Could you check a few things on this model? Use its own coordinates, in mm. Face numbers are marked on the shaded views. A direction names the side the tool comes from. Give positions to 0.01 mm unless a question says otherwise; leave off trailing zeros. Loops run counter-clockwise (first coordinate to the right, second up) from the corner with the lowest first, then second, coordinate; pieces in that order, holes last. Notation, with made-up numbers: M -3,-22 L 38,-22 A22 ccw 38,11 Z; hole C 23.25,16.25 d4. An arc over 180 degrees is marked long. Use CSV: the item, a comma, the result in double quotes.
```python
from build123d import *

# Parameters (mm, degrees)
F0_R     = 3.175
F1_DEPTH = 6.35
F2_R     = 1.8288
F3_R     = 1.8288
F4_DEPTH = 6.005883
F5_R     = 2.54


with BuildPart() as f1:
    # F0 (on Top) → F1 (new body)
    with BuildSketch(Plane.XY):
        with BuildLine():
            ThreePointArc((0, 13.335), (13.335, 0), (0, -13.335))
            Line((0, -13.335), (0, -31.446429))
            Line((0, -31.446429), (6.005883, -31.446429))
            Line((6.005883, -31.446429), (6.005883, -18.746429))
            ThreePointArc((6.005883, -18.746429), (14.263495, -13.566575), (19.023542, -5.060048))
            ThreePointArc((19.023542, -5.060048), (29.21, 0), (19.023542, 5.060048))
            ThreePointArc((19.023542, 5.060048), (14.263495, 13.566575), (6.005883, 18.746429))
            Line((6.005883, 18.746429), (6.005883, 31.446429))
            Line((6.005883, 31.446429), (0, 31.446429))
            Line((0, 31.446429), (0, 13.335))
        make_face()
        with Locations((22.86, 0)):
            Circle(F0_R, mode=Mode.SUBTRACT)
    extrude(amount=F1_DEPTH)

    # F2 (on face) + F3 (on face) → F4 (cut, through all)
    with BuildSketch(Plane.YZ.offset(6.005883)):
        with Locations((-25.096429, 3.175)):
            Circle(F2_R)
    with BuildSketch(Plane.YZ.offset(6.005883)):
        with Locations((25.096429, 3.175)):
            Circle(F3_R)
    extrude(amount=-F4_DEPTH, mode=Mode.SUBTRACT)

    # F5
    f5_edges = [f1.edges().sort_by_distance(p)[0] for p in [
        (19.023542, 5.060048, 3.175),
        (19.023542, -5.060048, 3.175),
        (6.005883, -18.746429, 3.175),
        (6.005883, 18.746429, 3.175),
    ]]
    fillet(f5_edges, radius=F5_R)


solid = f1.part
```
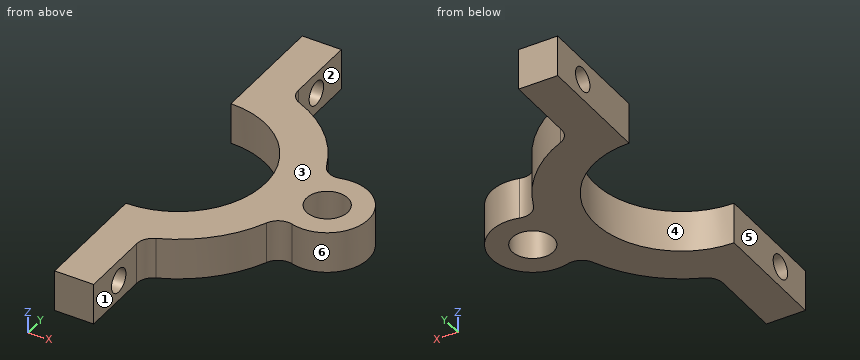
1. I'm going to push flat-ended pins straight in: pin 1 Ø1.5 at (x, z) = (20, 1.5) entering from -Y; pin 2 Ø1.9 at (y, z) = (24, 3) entering from +X; pin 3 Ø2 at (x, y) = (6, 9.5) entering from +Z; pin 4 Ø3 at (x, z) = (9, 4) entering from +Y. Where does each tip first touch, or does it pass through?
Outcome:
pin 1,"y = -6.36"
pin 2,"x = 6.01"
pin 3,"through"
pin 4,"y = 18.2"
2. Which directions (+Z, -Z, +X, -X, +Y, -Y) give clear straight access to the entire face, cutting with the end or side of a thin tool? Please do the marked faces 1, 2 and 3.
Outcome:
face 1,"+Z, -Z, +X, -Y"
face 2,"+Z, -Z, +X, +Y"
face 3,"+Z, +X, -X, +Y, -Y"
3. I want a section at D-D, the plane x = 16. List the corners of the cut face in (y, z) for me.
Outcome:
outline,"M -11.47,0 L 11.47,0 L 11.47,6.35 L -11.47,6.35 Z"
4. I want a section at C-C, the plane y = -28. List the corners of the cut face in (x, z) for me, then the cut area to 3 significant figures.
Outcome:
outline,"M 0,0 L 6.01,0 L 6.01,6.35 L 0,6.35 Z"
area,"38.1 mm2"
5. Please list where these lines run through material, in increasing order: line 1 (Y direction, x = 22.86, z = 4.25) (3 decimals); line 2 (Y direction, x = 1, z = 2); line 3 (Y direction, x = 4.5, z = 6).
Outcome:
line 1,"-6.35 to -3.175, 3.175 to 6.35"
line 2,"-31.45 to -26.5, -23.7 to -13.3, 13.3 to 23.7, 26.5 to 31.45"
line 3,"-31.45 to -12.55, 12.55 to 31.45"
6. If we mould it in two halves opening along Y, with no side actions, what happens to the marked faces 4, 5 and 6? For each: +Y half, -Y half, draft (parallel to the pull), parting line (faces both ways), or undercut.
Outcome:
face 4,"undercut"
face 5,"draft"
face 6,"parting line"
7. I want a section at B-B, the plane y = 0. List the corners of the cut face in (x, z) for me (3 decimals), then the cut area to 3 significant figures.
Outcome:
outline,"M 13.335,0 L 19.685,0 L 19.685,6.35 L 13.335,6.35 Z; M 26.035,0 L 29.21,0 L 29.21,6.35 L 26.035,6.35 Z"
area,"60.5 mm2"
8. I want a section at A-A, the plane x = 22.86. List the corners of the cut face in (y, z) for me (3 decimals), then the cut area to 3 significant figures.
Outcome:
outline,"M -6.35,0 L -3.175,0 L -3.175,6.35 L -6.35,6.35 Z; M 3.175,0 L 6.35,0 L 6.35,6.35 L 3.175,6.35 Z"
area,"40.3 mm2"
